Input: part model. Units: mm. Frame: model coordinates. A direction names the side the tool comes from. Give positions to 0.01 mm unless a question says otherwise; leave off trailing zeros. Loops run counter-clockwise (first coordinate to the right, second up) from the corner with the lowest first, then second, coordinate; pieces in that order, holes last.
from build123d import *

# Parameters (mm, degrees)
ESQUISSE1_W                     = 250
ESQUISSE1_H                     = 400
BOSS_EXTRU_1_DEPTH              = 10
ESQUISSE2_R                     = 13.5
ENL_V_MAT_EXTRU_1_DEPTH         = 237.061432682
CHANFREIN1_SIZE                 = 3
TROU_TARAUD_M51_D               = 4.2
TROUS_DE_CENTRAGE_4_0MM2_D      = 4
TROUS_DE_CENTRAGE_6_0MM2_D      = 6
D_GAGEMENT_M41_D                = 4.5
R_P_TITION_LIN_AIRE1_COUNT      = 2
R_P_TITION_LIN_AIRE1_PITCH      = 120
R_P_TITION_LIN_AIRE1_COUNT_DIR2 = 2
R_P_TITION_LIN_AIRE1_PITCH_DIR2 = 340
R_P_TITION_LIN_AIRE2_COUNT      = 2
R_P_TITION_LIN_AIRE2_PITCH      = 30
R_P_TITION_LIN_AIRE2_COUNT_DIR2 = 2
R_P_TITION_LIN_AIRE2_PITCH_DIR2 = 25
R_P_TITION_LIN_AIRE3_COUNT      = 2
R_P_TITION_LIN_AIRE3_PITCH      = 120
R_P_TITION_LIN_AIRE3_COUNT_DIR2 = 2
R_P_TITION_LIN_AIRE3_PITCH_DIR2 = 340


with BuildPart() as part:
    # Esquisse1 → Boss.-Extru.1 (new body)
    with BuildSketch(Plane.XY):
        Rectangle(ESQUISSE1_W, ESQUISSE1_H)
    extrude(amount=BOSS_EXTRU_1_DEPTH)

    # Esquisse2 → Enlèv. mat.-Extru.1 (cut, through all)
    with BuildSketch(Plane(origin=(0, 0, 0), x_dir=(-1, 0, 0), z_dir=(0, 0, -1))):
        Circle(ESQUISSE2_R)
    extrude(amount=-ENL_V_MAT_EXTRU_1_DEPTH, mode=Mode.SUBTRACT)

    # Chanfrein1
    chanfrein1_edges = [part.edges().sort_by_distance(p)[0] for p in [
        (125, -200, 5),
        (-125, -200, 5),
        (-125, 200, 5),
        (125, 200, 5),
    ]]
    chamfer(chanfrein1_edges, length=CHANFREIN1_SIZE)

    # Trou taraudé M51 (through all)
    with Locations(Plane.XY.offset(10)):
        with Locations((-72.698486264, -161.07971462), (-72.698486264, -181.838730229), (-111.937151978, -181.838730229), (-111.937151978, -161.07971462)):
            Hole(TROU_TARAUD_M51_D / 2)

    # Trous de centrage Ø4.0mm2 (through all)
    with Locations(Plane.XY.offset(10)):
        with Locations((-93.86308218, -161.07971462), (-93.86308218, -181.838730229)):
            Hole(TROUS_DE_CENTRAGE_4_0MM2_D / 2)

    # Trous de centrage Ø6.0mm2 (through all)
    with Locations(Plane.XY.offset(10)):
        with Locations((16.357059687, 37.86831259), (37.86831259, -16.357059687), (-16.357059687, -37.86831259), (-37.86831259, 16.357059687)):
            Hole(TROUS_DE_CENTRAGE_6_0MM2_D / 2)

    # Dégagement M41 (through all)
    with Locations(Plane(origin=(0, 0, 0), x_dir=(-1, 0, 0), z_dir=(0, 0, -1))):
        with Locations((28, -187), (28, -157), (53, -157), (53, -187)):
            d_gagement_m41 = Hole(D_GAGEMENT_M41_D / 2)

    # Répétition linéaire1: D_gagement M41 2 × 2
    with Locations(*[(i * R_P_TITION_LIN_AIRE1_PITCH, j * R_P_TITION_LIN_AIRE1_PITCH_DIR2, 0) for i in range(R_P_TITION_LIN_AIRE1_COUNT) for j in range(R_P_TITION_LIN_AIRE1_COUNT_DIR2) if (i, j) != (0, 0)]):
        add(d_gagement_m41, mode=Mode.SUBTRACT)

    # Esquisse29 → Chambrage pour vis à tête ronde bombée M41 (revolve, cut)
    with BuildSketch(Plane(origin=(92, -157, 10), x_dir=(0, -1, 0), z_dir=(1, 0, 0))):
        Polygon((0, 0), (0, 10), (2.25, 10), (2.25, 3.125), (2.275, 3.1), (4.5, 3.1), (4.5, 0), align=None)
    chambrage_pour_vis_t_te_ronde_bomb_e_m = revolve(axis=Axis((92, -157, 16.35), (0, 0, -1)), mode=Mode.SUBTRACT)

    # Répétition linéaire2: Chambrage pour vis _ t_te ronde bomb_e M 2 × 2
    with Locations(*[(-j * R_P_TITION_LIN_AIRE2_PITCH_DIR2, -i * R_P_TITION_LIN_AIRE2_PITCH, 0) for i in range(R_P_TITION_LIN_AIRE2_COUNT) for j in range(R_P_TITION_LIN_AIRE2_COUNT_DIR2) if (i, j) != (0, 0)]):
        add(chambrage_pour_vis_t_te_ronde_bomb_e_m, mode=Mode.SUBTRACT)

    # Répétition linéaire3: Chambrage pour vis _ t_te ronde bomb_e M 2 × 2
    with Locations(*[(-i * R_P_TITION_LIN_AIRE3_PITCH, j * R_P_TITION_LIN_AIRE3_PITCH_DIR2, 0) for i in range(R_P_TITION_LIN_AIRE3_COUNT) for j in range(R_P_TITION_LIN_AIRE3_COUNT_DIR2) if (i, j) != (0, 0)]):
        add(chambrage_pour_vis_t_te_ronde_bomb_e_m, mode=Mode.SUBTRACT)

    # Répétition linéaire3 copy 1 sketch → Répétition linéaire3 copy 1 (revolve, cut)
    with BuildSketch(Plane(origin=(67, 183, 10), x_dir=(0, -1, 0), z_dir=(1, 0, 0))):
        Polygon((0, 0), (0, 10), (2.25, 10), (2.25, 3.125), (2.275, 3.1), (4.5, 3.1), (4.5, 0), align=None)
    revolve(axis=Axis((67, 183, 16.35), (0, 0, -1)), mode=Mode.SUBTRACT)

    # Répétition linéaire3 copy 2 sketch → Répétition linéaire3 copy 2 (revolve, cut)
    with BuildSketch(Plane(origin=(-53, -157, 10), x_dir=(0, -1, 0), z_dir=(1, 0, 0))):
        Polygon((0, 0), (0, 10), (2.25, 10), (2.25, 3.125), (2.275, 3.1), (4.5, 3.1), (4.5, 0), align=None)
    revolve(axis=Axis((-53, -157, 16.35), (0, 0, -1)), mode=Mode.SUBTRACT)

    # Répétition linéaire3 copy 3 sketch → Répétition linéaire3 copy 3 (revolve, cut)
    with BuildSketch(Plane(origin=(-53, 183, 10), x_dir=(0, -1, 0), z_dir=(1, 0, 0))):
        Polygon((0, 0), (0, 10), (2.25, 10), (2.25, 3.125), (2.275, 3.1), (4.5, 3.1), (4.5, 0), align=None)
    revolve(axis=Axis((-53, 183, 16.35), (0, 0, -1)), mode=Mode.SUBTRACT)

    # Répétition linéaire3 copy 4 sketch → Répétition linéaire3 copy 4 (revolve, cut)
    with BuildSketch(Plane(origin=(92, 153, 10), x_dir=(0, -1, 0), z_dir=(1, 0, 0))):
        Polygon((0, 0), (0, 10), (2.25, 10), (2.25, 3.125), (2.275, 3.1), (4.5, 3.1), (4.5, 0), align=None)
    revolve(axis=Axis((92, 153, 16.35), (0, 0, -1)), mode=Mode.SUBTRACT)

    # Répétition linéaire3 copy 5 sketch → Répétition linéaire3 copy 5 (revolve, cut)
    with BuildSketch(Plane(origin=(-28, -187, 10), x_dir=(0, -1, 0), z_dir=(1, 0, 0))):
        Polygon((0, 0), (0, 10), (2.25, 10), (2.25, 3.125), (2.275, 3.1), (4.5, 3.1), (4.5, 0), align=None)
    revolve(axis=Axis((-28, -187, 16.35), (0, 0, -1)), mode=Mode.SUBTRACT)

    # Répétition linéaire3 copy 6 sketch → Répétition linéaire3 copy 6 (revolve, cut)
    with BuildSketch(Plane(origin=(-28, 153, 10), x_dir=(0, -1, 0), z_dir=(1, 0, 0))):
        Polygon((0, 0), (0, 10), (2.25, 10), (2.25, 3.125), (2.275, 3.1), (4.5, 3.1), (4.5, 0), align=None)
    revolve(axis=Axis((-28, 153, 16.35), (0, 0, -1)), mode=Mode.SUBTRACT)

    # Répétition linéaire3 copy 7 sketch → Répétition linéaire3 copy 7 (revolve, cut)
    with BuildSketch(Plane(origin=(67, 153, 10), x_dir=(0, -1, 0), z_dir=(1, 0, 0))):
        Polygon((0, 0), (0, 10), (2.25, 10), (2.25, 3.125), (2.275, 3.1), (4.5, 3.1), (4.5, 0), align=None)
    revolve(axis=Axis((67, 153, 16.35), (0, 0, -1)), mode=Mode.SUBTRACT)

    # Répétition linéaire3 copy 8 sketch → Répétition linéaire3 copy 8 (revolve, cut)
    with BuildSketch(Plane(origin=(-53, -187, 10), x_dir=(0, -1, 0), z_dir=(1, 0, 0))):
        Polygon((0, 0), (0, 10), (2.25, 10), (2.25, 3.125), (2.275, 3.1), (4.5, 3.1), (4.5, 0), align=None)
    revolve(axis=Axis((-53, -187, 16.35), (0, 0, -1)), mode=Mode.SUBTRACT)

    # Répétition linéaire3 copy 9 sketch → Répétition linéaire3 copy 9 (revolve, cut)
    with BuildSketch(Plane(origin=(-53, 153, 10), x_dir=(0, -1, 0), z_dir=(1, 0, 0))):
        Polygon((0, 0), (0, 10), (2.25, 10), (2.25, 3.125), (2.275, 3.1), (4.5, 3.1), (4.5, 0), align=None)
    revolve(axis=Axis((-53, 153, 16.35), (0, 0, -1)), mode=Mode.SUBTRACT)


solid = part.part
(1) Mould query, pull axis X, two halves, no side actions, for faces 3 (the cylindrical face through (65.648, 148.708, 8.472)), 4 (the flat face through (-125, -3, 5)), 5 (the flat face through (125, -3, 5)). Classes: +X half, -X half, draft (parallel to the pull), parting line (faces both ways), or undercut.
Values follow:
face 3: undercut
face 4: -X half
face 5: +X half
(2) Reachability of faces 1 (the flat face through (-30, 3, 0)), 2 (the cylindrical face through (-26.28, -161.16, 8.47)) from +Z, -Z, +X, -X, +Y, -Y: full face, straight path, thin tool, end or side. Return the list, or none.
Values follow:
face 1: -Z, +X, -X, +Y, -Y
face 2: +Z
(3) Cut plane B-B (x = 0). Return the cut outline in (y, z), and give its area (3 significant figures).
Values follow:
outline: (-200, 0) - (-13.5, 0) - (-13.5, 10) - (-200, 10) - close; (13.5, 0) - (200, 0) - (200, 10) - (13.5, 10) - close
area: 3,730 mm2
(4) Pin query (flat end, axial travel): pin 1 Ø3.5 at (x, y) = (92, -187) entering from -Z; pin 2 Ø5.5 at (x, y) = (-28, -157) entering from +Z. Return the tip coordinate at first contact, or that it passes through.
Values follow:
pin 1: passes through
pin 2: stops at z = 6.9
(5) Ray query, probe 1 along Y at (x, z) = (-53, 8.3); probe 2 along X at (y, z) = (183, 7.8); probe 3 along Y at (x, z) = (-28, 2.75). Return the intervals inside material, ascending.
Values follow:
probe 1: y = -200 to -191.5, -182.5 to -161.5, -152.5 to 148.5, 157.5 to 178.5, 187.5 to 200
probe 2: x = -125 to -57.5, -48.5 to -32.5, -23.5 to 62.5, 71.5 to 87.5, 96.5 to 125
probe 3: y = -200 to -189.25, -184.75 to -159.25, -154.75 to 150.75, 155.25 to 180.75, 185.25 to 200
(6) Cut plane A-A (y = 0). Return the cut outline in (x, z).
Values follow:
outline: (-125, 0) - (-13.5, 0) - (-13.5, 10) - (-125, 10) - close; (13.5, 0) - (125, 0) - (125, 10) - (13.5, 10) - close
